```python
from build123d import *

# Parameters (mm, degrees)
SKETCH1_W           = 1498.6
SKETCH1_H           = 50.8
BOSS_EXTRUDE1_DEPTH = 25.4
CUT_EXTRUDE1_DEPTH  = 1498.6
CUT_EXTRUDE2_DEPTH  = 1499.869043646
CUT_EXTRUDE3_DEPTH  = 1498.6
CUT_EXTRUDE4_DEPTH  = 1498.6
CUT_EXTRUDE5_DEPTH  = 1499.869043646
CUT_EXTRUDE6_DEPTH  = 1499.869043646
CUT_EXTRUDE7_DEPTH  = 1498.6
CUT_EXTRUDE8_DEPTH  = 1498.6
SKETCH10_W          = 20.32
SKETCH10_H          = 45.72
CUT_EXTRUDE9_DEPTH  = 1499.869043646
DRAFT1_ANGLE        = 45
DRAFT2_ANGLE        = 45.000000005
DRAFT3_ANGLE        = 45
DRAFT4_ANGLE        = 45
DRAFT5_ANGLE        = 45
DRAFT6_ANGLE        = 44.999999995
SKETCH11_W          = 61.962293059
SKETCH11_H          = 88.678950317
CUT_EXTRUDE10_DEPTH = 1041.4


with BuildPart() as part:
    # Sketch1 → Boss-Extrude1 (new body)
    with BuildSketch(Plane(origin=(12.7, 0, 0), x_dir=(0, 0, -1), z_dir=(1, 0, 0))):
        Rectangle(SKETCH1_W, SKETCH1_H)
    extrude(amount=-BOSS_EXTRUDE1_DEPTH)

    # Sketch2 → Cut-Extrude1 (cut)
    with BuildSketch(Plane.XY.offset(749.3)):
        Polygon((0.0762, 25.4), (-0.0762, 25.4), (0.0762, 25.2476), align=None)
    extrude(amount=-CUT_EXTRUDE1_DEPTH, mode=Mode.SUBTRACT)

    # Sketch3 → Cut-Extrude2 (cut, through all)
    with BuildSketch(Plane.XY.offset(749.3)):
        Polygon((12.7, 12.6238), (12.7, 12.7762), (12.5476, 12.7762), align=None)
    extrude(amount=-CUT_EXTRUDE2_DEPTH, mode=Mode.SUBTRACT)

    # Sketch4 → Cut-Extrude3 (cut)
    with BuildSketch(Plane.XY.offset(749.3)):
        Polygon((12.7, -0.0762), (12.7, 0.0762), (12.5476, -0.0762), align=None)
    extrude(amount=-CUT_EXTRUDE3_DEPTH, mode=Mode.SUBTRACT)

    # Sketch5 → Cut-Extrude4 (cut)
    with BuildSketch(Plane.XY.offset(749.3)):
        Polygon((12.7, -12.7762), (12.7, -12.6238), (12.5476, -12.6238), align=None)
    extrude(amount=-CUT_EXTRUDE4_DEPTH, mode=Mode.SUBTRACT)

    # Sketch6 → Cut-Extrude5 (cut, through all)
    with BuildSketch(Plane.XY.offset(749.3)):
        Polygon((0.0762, -25.4), (-0.0762, -25.2476), (-0.0762, -25.4), align=None)
    extrude(amount=-CUT_EXTRUDE5_DEPTH, mode=Mode.SUBTRACT)

    # Sketch7 → Cut-Extrude6 (cut, through all)
    with BuildSketch(Plane.XY.offset(749.3)):
        Polygon((-12.7, -12.6238), (-12.7, -12.7762), (-12.5476, -12.7762), align=None)
    extrude(amount=-CUT_EXTRUDE6_DEPTH, mode=Mode.SUBTRACT)

    # Sketch8 → Cut-Extrude7 (cut)
    with BuildSketch(Plane.XY.offset(749.3)):
        Polygon((-12.7, 0.0762), (-12.7, -0.0762), (-12.5476, 0.0762), align=None)
    extrude(amount=-CUT_EXTRUDE7_DEPTH, mode=Mode.SUBTRACT)

    # Sketch9 → Cut-Extrude8 (cut)
    with BuildSketch(Plane.XY.offset(749.3)):
        Polygon((-12.7, 12.7762), (-12.7, 12.6238), (-12.5476, 12.6238), align=None)
    extrude(amount=-CUT_EXTRUDE8_DEPTH, mode=Mode.SUBTRACT)

    # Sketch10 → Cut-Extrude9 (cut, through all)
    with BuildSketch(Plane.XY.offset(749.3)):
        Rectangle(SKETCH10_W, SKETCH10_H)
    extrude(amount=-CUT_EXTRUDE9_DEPTH, mode=Mode.SUBTRACT)

    # Draft1
    draft1_faces = [part.faces().sort_by_distance(p)[0] for p in [
        (0.0762, 25.3238, 0),
    ]]
    draft(draft1_faces, Plane(origin=(-12.7, 25.4, -749.3), x_dir=(0, 0, 1), z_dir=(0, 1, 0)), DRAFT1_ANGLE)

    # Draft2
    draft2_faces = [part.faces().sort_by_distance(p)[0] for p in [
        (12.6238, 12.7762, 0),
    ]]
    draft(draft2_faces, Plane(origin=(12.7, 0, 0), x_dir=(0, 0, 1), z_dir=(1, 0, 0)), DRAFT2_ANGLE)

    # Draft3
    draft3_faces = [part.faces().sort_by_distance(p)[0] for p in [
        (-0.0762, -25.3238, 0),
    ]]
    draft(draft3_faces, Plane(origin=(-12.7, -25.4, 749.3), x_dir=(0, 0, -1), z_dir=(0, -1, 0)), DRAFT3_ANGLE)

    # Draft4
    draft4_faces = [part.faces().sort_by_distance(p)[0] for p in [
        (-12.6238, -12.7762, 0),
    ]]
    draft(draft4_faces, Plane(origin=(-12.7, 0, 0), x_dir=(0, 0, -1), z_dir=(-1, 0, 0)), DRAFT4_ANGLE)

    # Draft5
    draft5_faces = [part.faces().sort_by_distance(p)[0] for p in [
        (12.6238, -12.6238, 0),
        (12.6238, 0, 0),
    ]]
    draft(draft5_faces, Plane(origin=(12.7, 0, 0), x_dir=(0, 0, 1), z_dir=(1, 0, 0)), DRAFT5_ANGLE)

    # Draft6
    draft6_faces = [part.faces().sort_by_distance(p)[0] for p in [
        (-12.6238, 0, 0),
        (-12.6238, 12.6238, 0),
    ]]
    draft(draft6_faces, Plane(origin=(-12.7, 0, 0), x_dir=(0, 0, -1), z_dir=(-1, 0, 0)), DRAFT6_ANGLE)

    # Sketch11 → Cut-Extrude10 (cut)
    with BuildSketch(Plane(origin=(0, 0, -749.3), x_dir=(-1, 0, 0), z_dir=(0, 0, -1))):
        with Locations((-2.92473676, 0.325700182)):
            Rectangle(SKETCH11_W, SKETCH11_H)
    extrude(amount=-CUT_EXTRUDE10_DEPTH, mode=Mode.SUBTRACT)


solid = part.part
```
Check sheet for the modelled part. Datum: model origin and axes. Units: mm. A direction names the side the tool comes from. Give positions to 0.01 mm unless a question says otherwise; leave off trailing zeros. Loops run counter-clockwise (first coordinate to the right, second up) from the corner with the lowest first, then second, coordinate; pieces in that order, holes last. Notation, with made-up numbers: M -22,59.5 L 5,59.5 A15 ccw 5,82.5 Z; hole C -9,36 d6. An arc over 180 degrees is marked long. Answer in a Markdown table with one row per item.
1) Cross-section at B-B (y = 17). Enter the section's corners in (x, z).
Solutions:
| item | result |
|---|---|
| outline | M -12.7,292.1 L -10.16,292.1 L -10.16,749.3 L -12.7,749.3 Z; M 10.16,292.1 L 12.7,292.1 L 12.7,749.3 L 10.16,749.3 Z |
2) Tool access check on faces 5 (the face through (10.16, 0, 524)), 6 (the face through (-12.7, 6, 524)). Record the directions out of +Z, -Z, +X, -X, +Y, -Y that give a thin tool (end or side, any length) a straight path to the whole face; none if there is none.
Solutions:
| item | result |
|---|---|
| face 5 | +Z, -Z |
| face 6 | +Z, -Z, -X, +Y, -Y |
3) Thickness scan on line 1 (Y direction, x = -3.75, z = 358.5); line 2 (X direction, y = -1.5, z = 464.5). Record the ranges inside material, lowest first.
Solutions:
| item | result |
|---|---|
| line 1 | y = -25.4 to -22.86, 22.86 to 25.4 |
| line 2 | x = -12.7 to -10.16, 10.16 to 12.7 |
4) Mould release check, pull along Y, two halves, no side actions. Record for faces 1 (the face through (0, 22.86, 524)), 2 (the face through (-6, 25.4, 524)), 3 (the face through (0, -22.86, 524)), 4 (the face through (12.7, 19, 524)): released by +Y, released by -Y, zero draft, split by the parting line, or undercut.
Solutions:
| item | result |
|---|---|
| face 1 | undercut |
| face 2 | released by +Y |
| face 3 | undercut |
| face 4 | zero draft |
5) Cross-section at A-A (x = 6.25). Enter the section's corners in (y, z), plus the area to 3 significant figures.
Solutions:
| item | result |
|---|---|
| outline | M -25.4,292.1 L -22.86,292.1 L -22.86,749.3 L -25.4,749.3 Z; M 22.86,292.1 L 25.4,292.1 L 25.4,749.3 L 22.86,749.3 Z |
| area | 2,320 mm^2 |
